The listing builds one solid part. Answer for the finished solid, in the listing's coordinates (mm). A direction names the side the tool comes from. Give positions to 0.01 mm unless a question says otherwise; leave off trailing zeros. Loops run counter-clockwise (first coordinate to the right, second up) from the corner with the lowest first, then second, coordinate; pieces in that order, holes last. Notation, with made-up numbers: (12.25, 56) - (54.25, 56) arc R23 ccw to (54.25, 91) - close; hole circle Ø2 at (2.25, -4.75). An arc over 180 degrees is marked (long way). Write each question's results on one line, items separated by ' | '.
from build123d import *

# Parameters (mm, degrees)
F1_DEPTH  = 20
F2_SIZE   = 10
F4_D      = 10
F4_DEPTH  = 100
F4_TIP    = 3.0043030951
F7_D      = 30
F7_DEPTH  = 100
F7_TIP    = 9.0129092854
F9_DEPTH  = 25
F10_R     = 2.5
F11_R     = 30
F12_R     = 1.4529244662
F12_R_2   = 3.4937424226
F12_R_3   = 7.4684037046
F13_DEPTH = 25
F15_D     = 7
F15_DEPTH = 100
F15_TIP   = 2.1030121666


with BuildPart() as f1:
    # F0 (on Top) → F1 (new body)
    with BuildSketch(Plane.XY):
        Polygon((75, -44.9038105677), (0, 85), (-75, -44.9038105677), align=None)
    extrude(amount=F1_DEPTH)

    # F2
    f2_edges = [f1.edges().sort_by_distance(p)[0] for p in [
        (-75, -44.903811, 10),
        (75, -44.903811, 10),
        (0, 85, 10),
    ]]
    chamfer(f2_edges, length=F2_SIZE)

    # F4
    with Locations(Plane.XY.offset(20)):
        with Locations((0, 60.3995919228), (52.3075809833, -30.1997959614), (-52.3075809833, -30.1997959614)):
            Hole(F4_D / 2, depth=F4_DEPTH)
            with Locations((0, 0, -(F4_DEPTH + F4_TIP / 2))):  # 118° drill point
                Cone(0, F4_D / 2, F4_TIP, mode=Mode.SUBTRACT)

    # F7
    with Locations(Plane.XY.offset(20)):
        with Locations((0, 0)):
            Hole(F7_D / 2, depth=F7_DEPTH)
            with Locations((0, 0, -(F7_DEPTH + F7_TIP / 2))):  # 118° drill point
                Cone(0, F7_D / 2, F7_TIP, mode=Mode.SUBTRACT)

    # F8 (on face) → F9 (cut)
    with BuildSketch(Plane.XY.offset(20)):
        Polygon((40, -34), (0, -24), (0, -48), (40, -48), align=None)
        Polygon((0, -48), (0, -24), (-40, -34), (-40, -48), align=None)
        Polygon((49.4448637287, -16.6410161514), (61.5692193817, -9.6410161514), (41.5692193817, 25), (20.7846096908, 13), align=None)
        Polygon((20.7846096908, 13), (41.5692193817, 25), (21.5692193817, 59.6410161514), (9.4448637287, 52.6410161514), align=None)
        Polygon((-10.3108891325, 52.1410161514), (-22.4352447854, 59.1410161514), (-42.4352447854, 24.5), (-21.6506350946, 12.5), align=None)
        Polygon((-21.6506350946, 12.5), (-42.4352447854, 24.5), (-62.4352447854, -10.1410161514), (-50.3108891325, -17.1410161514), align=None)
    extrude(amount=-F9_DEPTH, mode=Mode.SUBTRACT)

    # F10
    f10_edges = [f1.edges().sort_by_distance(p)[0] for p in [
        (-40, -34, 10),
        (-50.310889, -17.141016, 10),
        (-10.310889, 52.141016, 10),
        (9.444864, 52.641016, 10),
        (49.444864, -16.641016, 10),
        (40, -34, 10),
        (40, -44.903811, 10),
        (56.373067, -12.641016, 10),
        (16.373067, 56.641016, 10),
        (-16.80608, 55.891016, 10),
        (-56.80608, -13.391016, 10),
        (-40, -44.903811, 10),
    ]]
    fillet(f10_edges, radius=F10_R)

    # F11
    f11_edges = [f1.edges().sort_by_distance(p)[0] for p in [
        (0, -24, 10),
        (20.78461, 13, 10),
        (-21.650635, 12.5, 10),
    ]]
    fillet(f11_edges, radius=F11_R)

    # F12 (on face) → F13 (cut)
    with BuildSketch(Plane.XY.offset(20)):
        with Locations((0, 50)):
            Circle(F12_R)
        with Locations((0, 40)):
            Circle(F12_R_2)
        with Locations((0, 25)):
            Circle(F12_R_3)
        with Locations((-34.6410161514, -20)):
            Circle(F12_R_2)
        with Locations((-21.6506350946, -12.5)):
            Circle(F12_R_3)
        with Locations((-43.3012701892, -25)):
            Circle(F12_R)
        with Locations((34.6410161514, -20)):
            Circle(F12_R_2)
        with Locations((21.6506350946, -12.5)):
            Circle(F12_R_3)
        with Locations((43.3012701892, -25)):
            Circle(F12_R)
    extrude(amount=-F13_DEPTH, mode=Mode.SUBTRACT)

    # F15 (one way)
    with BuildSketch(Plane(origin=(0, 0, 0), x_dir=(1, 0, 0), z_dir=(0, 1, 0))):
        with Locations((0, -10.0512299687)):
            Circle(F15_D / 2)
    extrude(amount=-F15_DEPTH, mode=Mode.SUBTRACT)
    with Locations(Plane(origin=(0, 0, 0), x_dir=(1, 0, 0), z_dir=(0, 1, 0))):
        with Locations((0, -10.0512299687)):
            with Locations((0, 0, -(F15_DEPTH + F15_TIP / 2))):  # 118° drill point
                Cone(0, F15_D / 2, F15_TIP, mode=Mode.SUBTRACT)


solid = f1.part
Item 1: For faces 1 (the face through (12.693, 54.516, 10.14)), 2 (the face through (55.99, -26.82, 9.86)), 3 (the face through (-40, -39, 10)), 4 (the face through (-15.28, 34.77, 10.14)), determine the directions among +Z, -Z, +X, -X, +Y, -Y from which every point of the face is accessible in a straight line to the end or side of a thin tool.
Values found:
face 1: +Z, -Z, +X | face 2: +Z, -Z | face 3: +Z, -Z, -Y | face 4: +Z, -Z, -X
Item 2: A cutting plane is placed at C-C, the plane y = 25. Determine the outline of the cut face in (x, z), plus the area to 3 significant figures.
Values found:
outline: (-18.07, 0) - (-7.47, 0) - (-7.47, 20) - (-18.07, 20) - close; (7.47, 0) - (17.35, 0) - (17.35, 20) - (7.47, 20) - close | area: 410 mm²
Item 3: A cutting plane is placed at A-A, the plane y = 0. Determine the outline of the cut face in (x, z), plus the area to 3 significant figures.
Values found:
outline: (-33.74, 0) - (-15, 0) - (-15, 20) - (-33.74, 20) - close; (15, 0) - (33.35, 0) - (33.35, 20) - (15, 20) - close | area: 742 mm²
Item 4: Flat-ended cylindrical pins translate along their axes: P1, Ø2.5, axis at x = -43.3, y = -25, coming from the -Z side; P2, Ø8, axis at y = 30.5, z = 4, coming from the +X side; P3, Ø7, axis at y = -39, z = 8.5, coming from the +X side; P4, Ø4, axis at y = 38, z = 12, coming from the +X side. Find the tip coordinate at first contact, or state that the pin passes through.
Values found:
P1: passes through | P2: stops at x = 16.92 | P3: stops at x = 70 | P4: stops at x = 14.21
Item 5: A cutting plane is placed at D-D, the plane y = 67.5. Determine the outline of the cut face in (x, z), plus the area to 3 significant figures.
Values found:
outline: (-10.1, 0) - (10.1, 0) - (10.1, 20) - (-10.1, 20) - close | area: 404 mm²
Item 6: For a pull along Z with two mould halves and no side action, classify faces 5 (the face through (-0.759, -19.782, 13.468)), 6 (the face through (-37.41, -22.13, 10.14)), 7 (the face through (-0.3, -15.4, 20)) as released by +Z, released by -Z, zero draft, split by the parting line, or undercut.
Values found:
face 5: undercut | face 6: zero draft | face 7: released by +Z
Item 7: A cutting plane is placed at B-B, the plane z = 2.5. Count the separate pieces of the cut face and the enclosed holes in it, plus the area to 3 significant figures.
Values found:
separate pieces: 1 | enclosed holes: 13 | area: 4,710 mm²
Item 8: Find the intervals of material crossed by line 1 along Y through (x, z) = (0, 7); line 2 along Z through (x, y) = (0, -21); line 3 along X through (y, z) = (29.5, 8), in increasing order. Write a range as [from, to].
Values found:
line 1: y = [15, 17.53], [32.47, 36.51], [43.49, 48.55], [51.45, 55.4], [65.4, 76.34] | line 2: z = [0, 6.55], [13.55, 20] | line 3: x = [-16.79, -5.96], [5.96, 16.06]
